Autodesk Inventor part; units mm, degrees
ref_plane "YZ Plane" through (0, 0, 0) normal (1, 0, 0) x (0, 1, 0)
ref_plane "XZ Plane" through (0, 0, 0) normal (0, 1, 0) x (-1, 0, 0)
ref_plane "XY Plane" through (0, 0, 0) normal (0, 0, 1) x (1, 0, 0)
sketch "Esboço1" plane through (0, 0, 0) normal (0, 0, 1) x (1, 0, 0)
  line L0 (0, 0) -> (60, 0)
  line L1 (60, 0) -> (60, 110)
  line L2 (60, 110) -> (0, 110)
  line L3 (0, 110) -> (0, 0)
  line L4 (62, 112) -> (62, -2)
  line L5 (62, -2) -> (-2, -2)
  line L6 (-2, -2) -> (-2, 112)
  line L7 (-2, 112) -> (62, 112)
  dimension "d0" = 60
  dimension "d1" = 110
  dimension "d2" = 2
extrude "Extrusão1" add sketch "Esboço1" along normal blind 2 contours L3 L2 L1 L0 | L4 L5 L6 L7
sketch "Esboço2" plane through (0, 0, 2) normal (0, 0, 1) x (1, 0, 0)
  line L0 (62, 112) -> (-2, 112)
  line L1 (-2, 112) -> (-2, -2)
  line L2 (62, -2) -> (62, 112)
  line L3 (-2, -2) -> (62, -2)
  line L4 (0, 0) -> (0, 110)
  line L5 (0, 110) -> (60, 110)
  line L6 (60, 110) -> (60, 0)
  line L7 (60, 0) -> (0, 0)
  point P0 (0, 0)
  dimension "d5" = 2
extrude "Extrusão2" add sketch "Esboço2" along normal blind 38
sketch "Esboço3" plane through (-2, -2, 0) normal (0, -1, 0) x (1, 0, 0)
  line L0 (32, 5) -> (42, 5)
  line L1 (42, 5) -> (42, 15)
  line L2 (42, 15) -> (32, 15)
  line L3 (32, 15) -> (32, 5)
  line L4 (0, 0) -> (64, 0)
  line L5 (64, 0) -> (64, 40)
  point P0 (2, 0)
  dimension "d8" = 10
  dimension "d9" = 10
  dimension "d10" = 5
  dimension "d11" = 22
extrude "Extrusão3" cut sketch "Esboço3" against normal blind 38
sketch "Esboço11" plane through (-2, 112, 0) normal (0, 1, 0) x (1, 0, 0)
  line L0 (64, 0) -> (64, -40)
  line L1 (0, 0) -> (64, 0)
  line L2 (64, 0) -> (64, -2)
  line L3 (64, -2) -> (0, -2)
  line L4 (0, -2) -> (0, 0)
  line L5 (64, 0) -> (0, 0)
  point P0 (2, 0)
  dimension "d45" = 2
  dimension "d46" = 0
  dimension "d47" = 64
extrude "Extrusão8" add sketch "Esboço11" along normal blind 32
sketch "Esboço12" plane through (-2, 112, 2) normal (0, 0, 1) x (1, 0, 0)
  line L0 (2, 7.5) -> (7, 7.5)
  line L1 (7, 7.5) -> (7, 22.5)
  line L2 (7, 22.5) -> (2, 22.5)
  line L3 (2, 22.5) -> (2, 7.5)
  line L4 (52, 7.5) -> (47, 7.5)
  line L5 (47, 7.5) -> (47, 22.5)
  line L6 (47, 22.5) -> (52, 22.5)
  line L7 (52, 22.5) -> (52, 7.5)
  line L8 (64, 0) -> (0, 0)
  line L9 (0, 0) -> (0, 32)
  point P0 (2, -112)
  dimension "d50" = 5
  dimension "d51" = 15
  dimension "d52" = 5
  dimension "d53" = 15
  dimension "d54" = 7.5
  dimension "d55" = 7.5
  dimension "d56" = 40
  dimension "d57" = 2
extrude "Extrusão9" add sketch "Esboço12" along normal blind 10
sketch "Esboço13" plane through (-2, 112, 2) normal (0, 0, 1) x (1, 0, 0)
  circle A0 centre (17, 15) radius 1.5
  circle A1 centre (17, 15) radius 2
  circle A2 centre (17, 15) radius 3.5
  line L0 (7, 7.5) -> (7, 22.5)
  line L1 (0, 32) -> (64, 32)
  point P0 (2, -112)
  dimension "d60" = 3
  dimension "d61" = 4
  dimension "d62" = 7
  dimension "d69" = 10
  dimension "d70" = 17
extrude "Extrusão10" add sketch "Esboço13" along normal blind 3 contours A2
fillet "Arredondamento1" radius 3.5 1 edges at (13, 127, 5)
sketch "Esboço14" plane through (15, 127, 2) normal (0, 0, 1) x (1, 0, 0)
  circle A0 centre (0, 0) radius 1.5
  point P0 (-15, -127)
  dimension "d66" = 3
extrude "Extrusão11" cut sketch "Esboço14" against normal blind 3
sketch "Esboço16" plane through (-2, 112, 2) normal (0, 0, 1) x (1, 0, 0)
  line L0 (47, 22.5) -> (47, 7.5)
  line L1 (7, 6.5) -> (47, 6.5)
  line L2 (47, 6.5) -> (47, 8.5)
  line L3 (47, 8.5) -> (7, 8.5)
  line L4 (7, 8.5) -> (7, 6.5)
  line L5 (7, 7.5) -> (7, 22.5)
  line L6 (47, 23.5) -> (7, 23.5)
  line L7 (7, 23.5) -> (7, 21.5)
  line L8 (7, 21.5) -> (47, 21.5)
  line L9 (47, 21.5) -> (47, 23.5)
  circle A0 centre (17, 15) radius 1.5
  point P0 (2, -112)
  point P1 (47, 21.5)
  dimension "d77" = 2
  dimension "d78" = 2
  dimension "d79" = 13
  dimension "d80" = 6.5
  dimension "d81" = 40
extrude "Extrusão13" add sketch "Esboço16" along normal blind 10 contours L0 L8 L5 L7 L6 L9 | L0 L2 L1 L4 L3
sketch "Esboço17" plane through (5, 133.5, 2) normal (0, 0, 1) x (1, 0, 0)
  line L0 (0, 0) -> (40, 0)
  line L1 (23.5, 0) -> (21.5, 0)
  line L2 (21.5, 0) -> (21.5, -13)
  line L3 (21.5, -13) -> (23.5, -13)
  line L4 (23.5, -13) -> (23.5, 0)
  line L5 (40, -13) -> (0, -13)
  circle A0 centre (10, -6.5) radius 1.5
  point P0 (-5, -133.5)
  point P1 (21.5, 0)
  dimension "d84" = 0
  dimension "d85" = 2
  dimension "d86" = 10
extrude "Extrusão14" add sketch "Esboço17" along normal blind 10 contours L0 L4 L3 L2
sketch "Esboço18" plane through (-2, 112, 2) normal (0, 0, 1) x (1, 0, 0)
  line L0 (30.5, 21.5) -> (30.5, 8.5)
  line L1 (30.5, 8.5) -> (47, 8.5)
  line L2 (47, 8.5) -> (47, 21.5)
  line L3 (47, 21.5) -> (30.5, 21.5)
  line L4 (28.5, 8.5) -> (28.5, 21.5)
  line L5 (28.5, 21.5) -> (7, 21.5)
  line L6 (7, 21.5) -> (7, 8.5)
  line L7 (7, 8.5) -> (28.5, 8.5)
  circle A0 centre (17, 15) radius 1.5
  circle A1 centre (17, 15) radius 2
  circle A2 centre (17, 15) radius 3.5
  line L8 (52, 22.5) -> (52, 7.5)
  line L9 (52, 7.5) -> (47, 7.5)
  line L10 (47, 7.5) -> (47, 6.5)
  line L11 (47, 6.5) -> (7, 6.5)
  line L12 (7, 6.5) -> (7, 7.5)
  line L13 (7, 7.5) -> (2, 7.5)
  line L14 (2, 7.5) -> (2, 22.5)
  line L15 (2, 22.5) -> (7, 22.5)
  line L16 (7, 22.5) -> (7, 23.5)
  line L17 (7, 23.5) -> (47, 23.5)
  line L18 (47, 23.5) -> (47, 22.5)
  line L19 (47, 22.5) -> (52, 22.5)
  line L20 (0, 0) -> (64, 0)
  line L21 (64, 32) -> (64, 0)
  line L22 (0, 32) -> (64, 32)
  line L23 (0, 0) -> (0, 32)
  line L24 (0, -114) -> (0, 0)
  line L25 (64, -114) -> (0, -114)
  line L26 (64, 0) -> (64, -114)
  line L27 (2, -112) -> (62, -112)
  line L28 (62, -112) -> (62, -2)
  line L29 (62, -2) -> (2, -2)
  line L30 (2, -2) -> (2, -112)
  line L31 (62, 0) -> (62, 30)
  line L32 (62, 30) -> (2, 30)
  line L33 (2, 30) -> (2, 0)
  point P0 (2, 7.5)
  dimension "d89" = 2
extrude "Extrusão15" add sketch "Esboço18" along normal blind 38 contours L14 L33 L20 L23 L22 L21 L31 L32
sketch "Esboço19" plane through (62, -2, 40) normal (1, 0, 0) x (0, 0, -1)
  line L0 (30, 144) -> (0, 144)
  line L1 (0, 144) -> (0, 114)
  line L2 (0, 114) -> (30, 114)
  line L3 (30, 114) -> (30, 144)
  line L4 (40, 0) -> (40, 146)
  line L5 (40, 146) -> (0, 146)
  line L6 (0, 0) -> (0, 146)
  point P0 (40, 2)
  dimension "d92" = 10
  dimension "d93" = 2
  dimension "d94" = 0
  dimension "d95" = 30
extrude "Extrusão16" cut sketch "Esboço19" against normal blind 2
chamfer "Chanfro1" distance 1.5 angle 45 1 edges at (50, 127, 12)
sketch "Esboço20" plane through (-2, -2, 0) normal (-1, 0, 0) x (0, 0, 1)
  line L0 (25, 86) -> (15, 86)
  line L1 (15, 86) -> (15, 96)
  line L2 (15, 96) -> (25, 96)
  line L3 (25, 96) -> (25, 86)
  line L4 (0, 146) -> (40, 146)
  line L5 (0, 146) -> (0, 0)
  point P0 (0, 2)
  dimension "d101" = 10
  dimension "d102" = 10
  dimension "d103" = 50
  dimension "d104" = 15
extrude "Extrusão17" cut sketch "Esboço20" against normal blind 2
sketch "Esboço21" plane through (0, 0, 2) normal (0, 0, 1) x (1, 0, 0)
  point P0 (0, 0)
sketch "Esboço22" plane through (0, 0, 2) normal (0, 0, 1) x (1, 0, 0)
  line L0 (110.309, -33.0792) -> (-25.5735, -33.0792)
  line L1 (-25.5735, -33.0792) -> (-25.5735, 112)
  line L2 (-25.5735, 112) -> (110.309, 112)
  line L3 (110.309, 112) -> (110.309, -33.0792)
  line L4 (62, 112) -> (0, 112)
  point P0 (0, 0)
  dimension "d107" = 0
extrude "Extrusão18" cut sketch "Esboço22" along normal mid plane 100
sketch "Esboço23" plane through (50, 119.5, 2) normal (0, 0, 1) x (1, 0, 0)
  line L0 (12, 24.5) -> (-52, 24.5)
  line L1 (12, 22.5) -> (-50, 22.5)
  line L2 (-50, 22.5) -> (-50, 24.5)
  line L3 (-50, 24.5) -> (12, 24.5)
  line L4 (12, 24.5) -> (12, 22.5)
  point P0 (-50, -119.5)
extrude "Extrusão19" cut sketch "Esboço23" along normal mid plane 100
properties part number "basecaixa"
The listing builds one solid part. Answer for the finished solid, in the listing's coordinates (mm). A direction names the side the tool comes from. Give positions to 0.01 mm unless a question says otherwise; leave off trailing zeros. Write each loop counter-clockwise with the first axis right and the second up, starting at its lowest first coordinate (ties: lowest second). Pieces come first, ordered by that corner, then holes. Notation, with made-up numbers: (59.25, 7.5) - (96.25, 7.5) arc R22 cw to (96.25, 43.5) - close; hole circle Ø5 at (29, -30). An arc over 180 degrees is marked (long way). Use one line per item in the form item = value. Start each with the question number.
1) The mould has two halves that part along X. Classify faces 1 (the face through (-2, 128, 20)), 2 (the face through (16, 133.5, 7)), 3 (the face through (61, 127, 10)): pulls with the +X half, pulls with the -X half, needs draft (parallel to the pull), parting line crosses it, or undercut.
2) Find section B-B on x = 15. Determine the outline of the cut face in (y, z).
3) Find section A-A on z = 7.5. Determine the outline of the cut face in (x, y), plus the area to 3 significant figures.
4) Consider line 1 along Y through (x, z) = (38, 5); line 2 along X through (y, z) = (131.5, 21.5); line 3 along Z through (x, y) = (39, 135). Determine where each line is inside the solid, lowest interval first. Write a range as from..to.
5) A tool of negligible diameter and unlimited length cuts with its end or side. For faces 4 (the face through (28.5, 127, 7)), 5 (the face through (60, 127, 6)), 6 (the face through (3, 134.5, 7)), from which of +Z, -Z, +X, -X, +Y, -Y can it reach the whole face along a straight path? Write none if from no direction.
6) Flat-ended cylindrical pins translate along their axes: pin 1 Ø5 at (x, y) = (34, 125.5) entering from +Z; pin 2 Ø12 at (x, y) = (33, 139.5) entering from -Z; pin 3 Ø14.5 at (x, y) = (40.5, 124.5) entering from +Z; pin 4 Ø5 at (x, z) = (22, 7) entering from +Y. Find the tip coordinate at first contact, or state that the pin passes through.
7) Find section D-D on y = 115. Determine the outline of the cut face in (x, z), plus the area to 3 significant figures.
Geometry results:
q1.face_1 = pulls with the -X half
q1.face_2 = undercut
q1.face_3 = needs draft
q2.outline = (112, 0) - (125.5, 0) - (125.5, 2) - (125, 2) - (125, 2.13) arc R3.5 ccw to (123.5, 5) - (123.5, 2) - (120.5, 2) - (120.5, 12) - (118.5, 12) - (118.5, 2) - (112, 2) - close; (128.5, 0) - (142, 0) - (142, 2) - (135.5, 2) - (135.5, 12) - (133.5, 12) - (133.5, 2) - (130.5, 2) - (130.5, 5) arc R3.5 ccw to (129, 2.13) - (129, 2) - (128.5, 2) - close
q3.outline = (-2, 112) - (0, 112) - (0, 119.5) - (5, 119.5) - (5, 118.5) - (45, 118.5) - (45, 119.5) - (50, 119.5) - (50, 134.5) - (45, 134.5) - (45, 135.5) - (5, 135.5) - (5, 134.5) - (0, 134.5) - (0, 144) - (-2, 144) - close; (60, 112) - (62, 112) - (62, 142) - (60, 142) - close; hole (5, 120.5) - (26.5, 120.5) - (26.5, 133.5) - (5, 133.5) - close; hole (28.5, 120.5) - (45, 120.5) - (45, 133.5) - (28.5, 133.5) - close
q3.area = 460 mm2
q4.line_1 = 118.5..120.5, 133.5..135.5
q4.line_2 = -2..0
q4.line_3 = 0..12
q5.face_4 = +Z
q5.face_5 = +Z, +Y, -Y
q5.face_6 = +Z, +Y
q6.pin_1 = 2
q6.pin_2 = 0
q6.pin_3 = 12
q6.pin_4 = 135.5
q7.outline = (-2, 0) - (62, 0) - (62, 10) - (60, 10) - (60, 2) - (0, 2) - (0, 40) - (-2, 40) - close
q7.area = 220 mm2
